For this review, take the finished solid that the model builds, in its own axes (mm). A direction names the side the tool comes from. Round coordinates to 2 decimals unless told otherwise and drop trailing zeros. Order: outer loops, then holes, each group sorted by start corner. A loop starts at its lowest first (then second) coordinate and runs counter-clockwise, first axis right, second up. Notation, with made-up numbers: M -38,-12 L -8,-12 A25 cw -8,11 Z; hole C -16.5,85 d6. An arc over 180 degrees is marked long. Write item = value, one per line. Start each with the question number.
from build123d import *

# Parameters (mm, degrees)
F1_DEPTH = 25.4


with BuildPart() as f1:
    # F0 (on Front) → F1 (new body)
    with BuildSketch(Plane.XZ):
        with BuildLine():
            ThreePointArc((-9.525, 114.3), (-6.7351920908, 107.5648079092), (0, 104.775))
            ThreePointArc((0, 104.775), (6.7351920908, 107.5648079092), (9.525, 114.3))
            ThreePointArc((9.525, 114.3), (0, 123.825), (-9.525, 114.3))
        make_face()
        with BuildLine():
            ThreePointArc((6.104734078, 114.063590765), (4.3089160173, 109.7911312939), (0, 108.084639221))
            ThreePointArc((0, 108.084639221), (-4.0599425849, 118.3360502361), (6.104734078, 114.063590765))
        make_face(mode=Mode.SUBTRACT)
        with BuildLine():
            ThreePointArc((9.525, 114.3), (6.7351920908, 107.5648079092), (0, 104.775))
            Line((0, 104.775), (0, 103.7053296111))
            ThreePointArc((0, 103.7053296111), (0.6520493641, 102.6722677878), (0.8799784566, 101.4720872045))
            ThreePointArc((0.8799784566, 101.4720872045), (0.6520493641, 100.2719066211), (0, 99.2388447978))
            Line((0, 99.2388447978), (0, 79.375))
            ThreePointArc((0, 79.375), (10.4912828548, 75.4142187767), (15.7474569047, 65.5082893304))
            Line((15.7474569047, 65.5082893304), (9.525, 114.3))
        make_face()
        with BuildLine():
            Line((0, 103.7053296111), (0, 104.775))
            ThreePointArc((0, 104.775), (-6.7351920908, 107.5648079092), (-9.525, 114.3))
            Line((-9.525, 114.3), (-15.7474569047, 65.5082893304))
            ThreePointArc((-15.7474569047, 65.5082893304), (-10.4912828548, 75.4142187767), (0, 79.375))
            Line((0, 79.375), (0, 99.2388447978))
            ThreePointArc((0, 99.2388447978), (-5.6676065299, 101.4720872045), (0, 103.7053296111))
        make_face()
        with BuildLine():
            ThreePointArc((0, 79.375), (-10.4912828548, 75.4142187767), (-15.7474569047, 65.5082893304))
            ThreePointArc((-15.7474569047, 65.5082893304), (-15.875, 63.5), (-15.7474569047, 61.4917106696))
            ThreePointArc((-15.7474569047, 61.4917106696), (-10.4912828548, 51.5857812233), (0, 47.625))
            Line((0, 47.625), (0, 58.6328048089))
            ThreePointArc((0, 58.6328048089), (-4.8671951911, 63.5), (0, 68.3671951911))
            Line((0, 68.3671951911), (0, 79.375))
        make_face()
        with BuildLine():
            ThreePointArc((15.875, 63.5), (15.8430821396, 64.5061676396), (15.7474569047, 65.5082893304))
            ThreePointArc((15.7474569047, 65.5082893304), (10.4912828548, 75.4142187767), (0, 79.375))
            Line((0, 79.375), (0, 68.3671951911))
            ThreePointArc((0, 68.3671951911), (3.441626725, 66.941626725), (4.8671951911, 63.5))
            ThreePointArc((4.8671951911, 63.5), (3.441626725, 60.058373275), (0, 58.6328048089))
            Line((0, 58.6328048089), (0, 47.625))
            ThreePointArc((0, 47.625), (10.4912828548, 51.5857812233), (15.7474569047, 61.4917106696))
            ThreePointArc((15.7474569047, 61.4917106696), (15.8430821396, 62.4938323604), (15.875, 63.5))
        make_face()
        with BuildLine():
            ThreePointArc((0, 47.625), (-10.4912828548, 51.5857812233), (-15.7474569047, 61.4917106696))
            Line((-15.7474569047, 61.4917106696), (-9.525, 0))
            ThreePointArc((-9.525, 0), (-6.7351920908, 6.7351920908), (0, 9.525))
            Line((0, 9.525), (0, 47.625))
        make_face()
        with BuildLine():
            ThreePointArc((15.7474569047, 61.4917106696), (10.4912828548, 51.5857812233), (0, 47.625))
            Line((0, 47.625), (0, 9.525))
            ThreePointArc((0, 9.525), (0.3388863295, 9.5189695375), (0.6773435479, 9.500885786))
            Line((0.6773435479, 9.500885786), (6.104734078, 9.3076644033))
            Line((6.104734078, 9.3076644033), (10.451200974, 9.1529251528))
            Line((10.451200974, 9.1529251528), (15.7474569047, 61.4917106696))
        make_face()
        with BuildLine():
            ThreePointArc((0, 9.525), (-6.7351920908, 6.7351920908), (-9.525, 0))
            ThreePointArc((-9.525, 0), (-6.7351920908, -6.7351920908), (0, -9.525))
            Line((0, -9.525), (0.6773435479, -9.500885786))
            ThreePointArc((0.6773435479, -9.500885786), (6.9705567315, -6.4912990883), (9.525, 0))
            Line((9.525, 0), (3.3982770983, 0))
            ThreePointArc((3.3982770983, 0), (-2.4029447806, -2.4029447806), (0, 3.3982770983))
            Line((0, 3.3982770983), (0, 9.525))
        make_face()
        with BuildLine():
            Line((0.6773435479, -9.500885786), (0, -9.525))
            ThreePointArc((0, -9.525), (0.3388863295, -9.5189695375), (0.6773435479, -9.500885786))
        make_face()
        with BuildLine():
            Line((9.525, 0), (10.451200974, 9.1529251528))
            Line((10.451200974, 9.1529251528), (6.104734078, 9.3076644033))
            Line((6.104734078, 9.3076644033), (6.104734078, 7.3114873204))
            ThreePointArc((6.104734078, 7.3114873204), (8.627665301, 4.0359653682), (9.525, 0))
        make_face()
        with BuildLine():
            Line((44.7324052746, 7.9324746146), (10.451200974, 9.1529251528))
            Line((10.451200974, 9.1529251528), (9.525, 0))
            Line((9.525, 0), (36.5125, 0))
            ThreePointArc((36.5125, 0), (38.9380895153, 5.7116327839), (44.7324052746, 7.9324746146))
        make_face()
        with BuildLine():
            ThreePointArc((9.525, 0), (6.9705567315, -6.4912990883), (0.6773435479, -9.500885786))
            Line((0.6773435479, -9.500885786), (44.7324052746, -7.9324746146))
            ThreePointArc((44.7324052746, -7.9324746146), (38.9380895153, -5.7116327839), (36.5125, 0))
            Line((36.5125, 0), (9.525, 0))
        make_face()
        with BuildLine():
            ThreePointArc((52.3875, 0), (50.1616327839, 5.5119104847), (44.7324052746, 7.9324746146))
            ThreePointArc((44.7324052746, 7.9324746146), (38.9380895153, 5.7116327839), (36.5125, 0))
            ThreePointArc((36.5125, 0), (38.9380895153, -5.7116327839), (44.7324052746, -7.9324746146))
            ThreePointArc((44.7324052746, -7.9324746146), (50.1616327839, -5.5119104847), (52.3875, 0))
        make_face()
        with BuildLine():
            ThreePointArc((47.4750581285, 0.236410473), (43.305671032, -4.0495958985), (38.9063060284, 0))
            ThreePointArc((38.9063060284, 0), (43.0691705984, 4.5224168445), (47.4750581285, 0.236410473))
        make_face(mode=Mode.SUBTRACT)
    extrude(amount=F1_DEPTH)


solid = f1.part
(1) For line 1 along X through (y, z) = (-2.25, -1); line 2 along Z through (x, y) = (1.5, -14); line 3 along X through (y, z) = (-23.75, 118), list the stretches that pass through material, from the lowest coordinate up.
(2) Insertion check: pin 1 (3 mm diameter, centred on x = 6, y = -19, fed in from -Z); pin 2 (1.5 mm diameter, centred on y = -3.5, z = 36.5, fed in from +X); pin 3 (4 mm diameter, centred on x = 2.5, y = -21, fed in from -Z). Each pin has a flat end and moves straight along its axis. Give the tip position at first contact, or say it passes through.
(3) For faces 1 (the flat face through (0, -13, 6)), 2 (the cylindrical face through (-15.875, -12.522, 63.528)), 3 (the flat face through (13.062, -12.522, 34.956)), list the 3-axis set-ups (+Z, -Z, +X, -X, +Y, -Y) from which the entire face can be reached by the end or side of a thin tool; tool diameter is ignored.
(4) We need section D-D, the plane x = 33. Write out the cut boundary in (y, z).
(5) We need section B-B, the plane z = 112. Write out the cut boundary in (x, y), then the cut area to 3 significant figures.
(6) We need section C-C, the plane x = 14. Write out the cut boundary in (y, z).
(7) We need section A-A, the plane y = -14.5. State how many separate pieces and enclosed holes the cut face has, then the cut area to 3 significant figures.
(8) Draft analysis for pull direction X (two halves, no side actions). For faces 4 (the flat face through (3, -25.4, 43)), 5 (the cylindrical face through (8.6, -12.52, 4.09)), 6 (the cylindrical face through (0.209, -12.522, 123.823)), state which applies: released by +X, released by -X, zero draft, split by the parting line, or undercut.
Values:
q1.line_1 = -9.47 to -3.25, 3.25 to 39.08, 47.29 to 52.32
q1.line_2 = -9.47 to -3.05, 9.47 to 58.87, 68.13 to 108.24, 119.88 to 123.71
q1.line_3 = -8.78 to -4.38, 4.63 to 8.78
q2.pin_1 = -9.36
q2.pin_2 = 13.29
q2.pin_3 = -9.51
q3.face_1 = +Y, -Y
q3.face_2 = -X, +Y, -Y
q3.face_3 = +X, +Y, -Y
q4.outline = M -25.4,-8.35 L 0,-8.35 L 0,8.35 L -25.4,8.35 Z
q5.outline = M -9.82,-25.4 L -5.49,-25.4 L -5.49,0 L -9.82,0 Z; M 5.74,-25.4 L 9.82,-25.4 L 9.82,0 L 5.74,0 Z
q5.area = 214 mm²
q6.outline = M -25.4,-9.03 L 0,-9.03 L 0,9.03 L -25.4,9.03 Z; M -25.4,44.22 L 0,44.22 L 0,79.21 L -25.4,79.21 Z
q7.separate_pieces = 1
q7.enclosed_holes = 5
q7.area = 3,530 mm²
q8.face_4 = zero draft
q8.face_5 = undercut
q8.face_6 = split by the parting line
